Model file for the job. Use its own axes, mm. A direction names the side the tool comes from. Round coordinates to 2 decimals unless told otherwise and drop trailing zeros. Write each loop counter-clockwise with the first axis right and the second up, starting at its lowest first coordinate (ties: lowest second). Pieces come first, ordered by that corner, then holes. Notation, with made-up numbers: (-17, -4.5) - (29, -4.5) arc R11 cw to (29, 2.5) - close; hole circle Ø7 at (59.25, 31). An arc over 180 degrees is marked (long way). Answer as a JSON object with one key per item and string values. Group by question number.
from build123d import *

# Parameters (mm, degrees)
F0_R      = 7.5
F1_DEPTH  = 21
F2_R      = 9.5
F3_DEPTH  = 5
F5_D      = 6.35
F5_DEPTH  = 15
F5_TIP    = 1.9077324654
F7_D      = 2.5
F7_DEPTH  = 9.501
F8_R      = 7.5
F9_DEPTH  = 5
F10_R     = 4
F11_DEPTH = 10
F13_R     = 7.5
F13_R_2   = 6.5
F14_DEPTH = 1.5


with BuildPart() as f1:
    # F0 (on Top) → F1 (new body)
    with BuildSketch(Plane.XY):
        Circle(F0_R)
    extrude(amount=F1_DEPTH)

    # F2 (on Top) → F3 (join)
    with BuildSketch(Plane.XY):
        Circle(F2_R)
    extrude(amount=F3_DEPTH)

    # F5
    with Locations(Plane(origin=(0, 0, 0), x_dir=(1, 0, 0), z_dir=(0, 0, -1))):
        with Locations((0, 0)):
            Hole(F5_D / 2, depth=F5_DEPTH)
            with Locations((0, 0, -(F5_DEPTH + F5_TIP / 2))):  # 118° drill point
                Cone(0, F5_D / 2, F5_TIP, mode=Mode.SUBTRACT)

    # F7 (through all, one way)
    with BuildSketch(Plane(origin=(0, 0, 0), x_dir=(1, 0, 0), z_dir=(0, 1, 0))):
        with Locations((0, -2.5)):
            Circle(F7_D / 2)
    extrude(amount=-F7_DEPTH, mode=Mode.SUBTRACT)

    # F8 (on face) → F9 (join)
    with BuildSketch(Plane.XY.offset(21)):
        Circle(F8_R)
    extrude(amount=F9_DEPTH)

    # F10 (on face) → F11 (join)
    with BuildSketch(Plane.XY.offset(26)):
        Circle(F10_R)
    extrude(amount=F11_DEPTH)

    # F13 (on offset) → F14 (cut)
    with BuildSketch(Plane.XY.offset(21.5)):
        Circle(F13_R)
        Circle(F13_R_2, mode=Mode.SUBTRACT)
    extrude(amount=F14_DEPTH, mode=Mode.SUBTRACT)


solid = f1.part
(1) 3-axis set-ups, long thin cutter, end or side, ignore diameter. For faces 1 (the cylindrical face through (-0.16, -6.16, 1.26)), 2 (the cylindrical face through (-5.158, -3.955, 22.24)), 3 (the flat face through (1, 8, 5)), 4 (the flat face through (0, 0, 36)), 5 (the cylindrical face through (0.69, 3.1, 7.6)): which of +Z, -Z, +X, -X, +Y, -Y reach the whole face in a straight line?
(2) Pull direction Z, two halves, no side cores. Call faces 6 (the flat face through (3, -3, 26)), 7 (the cylindrical face through (-7.493, 0.33, 24.479)), 8 (the conical face through (-0.1, -0.5, 16.6)), 9 (the flat face through (-6, 3, 23)): pulls with the +Z half, pulls with the -Z half, needs draft (parallel to the pull), parting line crosses it, or undercut.
(3) Slice it at B-B (x = -7). Write the cut outline in (y, z), then the cut area to 3 significant figures.
(4) Drill centre lines: line 1 (Y direction, x = 0, z = 4.5) (3 decimals); line 2 (Z direction, x = -2.75, y = 6.5); line 3 (Y direction, x = 0, z = 6.5) (3 decimals). Where is each one in solid material? Low to high. Write a range as from..to.
(5) Slice it at C-C (y = 5). Write the cut outline in (x, z).
(6) Flat gauge pins, fed straight in: pin 1 (3 mm diameter, centred on y = -4, z = 30.5, fed in from +X); pin 2 (1 mm diameter, centred on y = -2.5, z = 29, fed in from +X); pin 3 (4 mm diameter, centred on y = -4, z = 32.5, fed in from -X). Where does each tip first touch, or does it go through?
(7) Slice it at A-A (y = -7). Write the cut outline in (x, z).
(8) Slice it at D-D (z = 28.5). Write the cut outline in (x, y), then the cut area to 3 significant figures.
Answer:
{
 "1": {"face 1": "-Y", "face 2": "none", "face 3": "+Z", "face 4": "+Z, +X, -X, +Y, -Y", "face 5": "-Z"},
 "2": {"face 6": "pulls with the +Z half", "face 7": "needs draft", "face 8": "pulls with the -Z half", "face 9": "undercut"},
 "3": {"outline": "(-6.42, 0) - (6.42, 0) - (6.42, 5) - (2.69, 5) - (2.69, 21.5) - (-2.69, 21.5) - (-2.69, 5) - (-6.42, 5) - close; (-2.69, 23) - (2.69, 23) - (2.69, 26) - (-2.69, 26) - close", "area": "169 mm²"},
 "4": {"line 1": "-9.5..-3.175, 3.175..9.5", "line 2": "0..21.5, 23..26", "line 3": "-7.5..-3.175, 3.175..7.5"},
 "5": {"outline": "(-8.08, 0) - (8.08, 0) - (8.08, 5) - (5.59, 5) - (5.59, 21.5) - (4.15, 21.5) - (4.15, 23) - (5.59, 23) - (5.59, 26) - (-5.59, 26) - (-5.59, 23) - (-4.15, 23) - (-4.15, 21.5) - (-5.59, 21.5) - (-5.59, 5) - (-8.08, 5) - close"},
 "6": {"pin 1": "x = 3.12", "pin 2": "x = 3.46", "pin 3": "x = -3.46"},
 "7": {"outline": "(-6.42, 0) - (6.42, 0) - (6.42, 5) - (2.69, 5) - (2.69, 21.5) - (-2.69, 21.5) - (-2.69, 5) - (-6.42, 5) - close; (-2.69, 23) - (2.69, 23) - (2.69, 26) - (-2.69, 26) - close; hole circle Ø2.5 at (0, 2.5)"},
 "8": {"outline": "circle Ø8 at (0, 0)", "area": "50.3 mm²"}
}
